Can you work these out from the model? Positions are in its coordinate system, mm. Round coordinates to 2 decimals unless told otherwise and drop trailing zeros. Loops run counter-clockwise (first coordinate to the right, second up) from the corner with the lowest first, then second, coordinate; pieces in that order, holes last. Notation, with made-up numbers: M -13.75,40.25 L 22.25,40.25 A17 ccw 22.25,44.25 Z; hole C -20,46 d9. An arc over 180 degrees is marked long. Return JSON: item names as keys, results as strings.
```python
from build123d import *

# Parameters (mm, degrees)
BOSS_EXTRUDE1_DEPTH = 1.5
CHAMFER1_SIZE       = 1.5
CHAMFER1_SIZE_2     = 2.5


with BuildPart() as part:
    # Sketch1 → Boss-Extrude1 (new body)
    with BuildSketch(Plane(origin=(0, 0, 0), x_dir=(1, 0, 0), z_dir=(0, 1, 0))):
        with BuildLine():
            Line((-35, 40), (35, 40))
            ThreePointArc((35, 40), (38.535533906, 38.535533906), (40, 35))
            Line((40, 35), (40, -35))
            ThreePointArc((40, -35), (38.535533906, -38.535533906), (35, -40))
            Line((35, -40), (-35, -40))
            ThreePointArc((-35, -40), (-38.535533906, -38.535533906), (-40, -35))
            Line((-40, -35), (-40, 35))
            ThreePointArc((-40, 35), (-38.535533906, 38.535533906), (-35, 40))
        make_face()
    extrude(amount=BOSS_EXTRUDE1_DEPTH)

    # Chamfer1
    # the kernel refuses this chamfer: 2.5, 1.5 mm, written as the material it takes off along each edge
    with BuildSketch(Plane(origin=(-35, 1.5, 35), x_dir=(0, 0, 1), z_dir=(1, 0, 0))) as chamfer1_piece_1:
        Polygon((5, CHAMFER1_SIZE), (5 - CHAMFER1_SIZE_2, 0), (5, 0), align=None)
    revolve(axis=Axis((-35, 1.5, 35), (0, -1, 0)), revolution_arc=90, mode=Mode.SUBTRACT)
    with BuildSketch(Plane(origin=(-40, 1.5, 35), x_dir=(-0.05518620705976808, -0.9984760801092615, 0), z_dir=(0, 0, -1)), Plane(origin=(-35, 1.5, -40), x_dir=(0, -0.9984760801092615, -0.05518620705976808), z_dir=(1, 0, 0)), Plane(origin=(35, 1.5, 40), x_dir=(0, -0.9984760801092615, 0.05518620705976808), z_dir=(-1, 0, 0)), Plane(origin=(40, 1.5, -35), x_dir=(0.05518620705976808, -0.9984760801092615, 0), z_dir=(0, 0, 1))) as chamfer1_piece_2:
        Polygon((CHAMFER1_SIZE * 0.998476080109, -CHAMFER1_SIZE * 0.0551862070598), (-CHAMFER1_SIZE_2 * 0.0551862070598, -CHAMFER1_SIZE_2 * 0.998476080109), (0, 0), align=None)
    extrude(amount=70, mode=Mode.SUBTRACT)
    with BuildSketch(Plane(origin=(-35, 1.5, -35), x_dir=(-1, 0, 0), z_dir=(0, 0, 1))) as chamfer1_piece_3:
        Polygon((5, CHAMFER1_SIZE), (5 - CHAMFER1_SIZE_2, 0), (5, 0), align=None)
    revolve(axis=Axis((-35, 1.5, -35), (0, -1, 0)), revolution_arc=90, mode=Mode.SUBTRACT)
    with BuildSketch(Plane(origin=(35, 1.5, -35), x_dir=(0, 0, -1), z_dir=(-1, 0, 0))) as chamfer1_piece_4:
        Polygon((5, CHAMFER1_SIZE), (5 - CHAMFER1_SIZE_2, 0), (5, 0), align=None)
    revolve(axis=Axis((35, 1.5, -35), (0, -1, 0)), revolution_arc=90, mode=Mode.SUBTRACT)
    with BuildSketch(Plane(origin=(35, 1.5, 35), x_dir=(1, 0, 0), z_dir=(0, 0, -1))) as chamfer1_piece_5:
        Polygon((5, CHAMFER1_SIZE), (5 - CHAMFER1_SIZE_2, 0), (5, 0), align=None)
    revolve(axis=Axis((35, 1.5, 35), (0, -1, 0)), revolution_arc=90, mode=Mode.SUBTRACT)


solid = part.part
```
Q1. If I drill on line 1 along X through (y, z) = (0.4, -9); line 2 along X through (y, z) = (1.35, -1); line 3 along Z through (x, y) = (-4.5, 1.1), over which ranges is the centre line in solid material (lowest first)?
Results:
{"line 1": "x = -39.33 to 39.33", "line 2": "x = -37.75 to 37.75", "line 3": "z = -38.17 to 38.17"}
Q2. Suppose I cut it at C-C, the plane z = 16.5. Please give me the cut outline in (x, y).
Results:
{"outline": "M -40,0 L 40,0 L 37.5,1.5 L -37.5,1.5 Z"}
Q3. Suppose I cut it at A-A, the plane y = 0.3. Please give me the cut outline in (x, z).
Results:
{"outline": "M -39.5,-35 A4.5 ccw -35,-39.5 L 35,-39.5 A4.5 ccw 39.5,-35 L 39.5,35 A4.5 ccw 35,39.5 L -35,39.5 A4.5 ccw -39.5,35 Z"}
Q4. Suppose I cut it at B-B, the plane x = 13. Please give me the cut outline in (y, z), plus the area to 3 significant figures.
Results:
{"outline": "M 0,-40 L 1.5,-37.5 L 1.5,37.5 L 0,40 Z", "area": "116 mm2"}
